Check sheet for the modelled part. Datum: model origin and axes. Units: mm. A direction names the side the tool comes from. Give positions to 0.01 mm unless a question says otherwise; leave off trailing zeros. Loops run counter-clockwise (first coordinate to the right, second up) from the corner with the lowest first, then second, coordinate; pieces in that order, holes last.
```python
from build123d import *

# Parameters (mm, degrees)
SKETCH1_W                    = 106
SKETCH1_H                    = 814
BASE_FLANGE1_DEPTH           = 1
EDGE_FLANGE1_STRIP_W         = 6
EDGE_FLANGE1_STRIP_H         = 1
EDGE_FLANGE1_STRIP_CUT_DEPTH = 814
EDGE_FLANGE1_DEPTH           = 814
EDGE_FLANGE2_STRIP_W         = 6
EDGE_FLANGE2_STRIP_H         = 1
EDGE_FLANGE2_STRIP_CUT_DEPTH = 814
EDGE_FLANGE2_DEPTH           = 814
EDGE_FLANGE4_STRIP_W         = 6
EDGE_FLANGE4_STRIP_H         = 1
EDGE_FLANGE4_STRIP_CUT_DEPTH = 814
EDGE_FLANGE4_DEPTH           = 814
SKETCH19_R                   = 3
CUT_EXTRUDE2_DEPTH           = 10


# Sheet-metal steps are written as plain solids
with BuildPart() as part:
    # Sketch1 → Base-Flange1 (new body)
    with BuildSketch(Plane(origin=(0, 0, 0), x_dir=(1, 0, 0), z_dir=(0, 1, 0))):
        with Locations((53, 407)):
            Rectangle(SKETCH1_W, SKETCH1_H)
    extrude(amount=-BASE_FLANGE1_DEPTH)

    # Edge-Flange1 strip (across the edge) → Edge-Flange1 strip cut (cut)
    with BuildSketch(Plane(origin=(106, 0, 0), x_dir=(-1, 0, 0), z_dir=(0, 0, -1))):
        with Locations((-1, -0.5)):
            Rectangle(EDGE_FLANGE1_STRIP_W, EDGE_FLANGE1_STRIP_H)
    extrude(amount=EDGE_FLANGE1_STRIP_CUT_DEPTH, mode=Mode.SUBTRACT)

    # Edge-Flange1 section (across the edge) → Edge-Flange1 (add)
    with BuildSketch(Plane(origin=(106, 0, 0), x_dir=(-1, 0, 0), z_dir=(0, 0, -1))):
        with BuildLine():
            Line((0, 1), (0, 19))
            Line((0, 19), (1, 19))
            Line((1, 19), (1, 1))
            ThreePointArc((1, 1), (1.292893219, 0.292893219), (2, 0))
            Line((2, 0), (2, -1))
            ThreePointArc((2, -1), (0.585786438, -0.414213562), (0, 1))
        make_face()
    extrude(amount=EDGE_FLANGE1_DEPTH)

    # Edge-Flange2 strip (across the edge) → Edge-Flange2 strip cut (cut)
    with BuildSketch(Plane(origin=(105, 19, 0), x_dir=(0, -1, 0), z_dir=(0, 0, -1))):
        with Locations((-1, -0.5)):
            Rectangle(EDGE_FLANGE2_STRIP_W, EDGE_FLANGE2_STRIP_H)
    extrude(amount=EDGE_FLANGE2_STRIP_CUT_DEPTH, mode=Mode.SUBTRACT)

    # Edge-Flange2 section (across the edge) → Edge-Flange2 (add)
    with BuildSketch(Plane(origin=(105, 19, 0), x_dir=(0, -1, 0), z_dir=(0, 0, -1))):
        with BuildLine():
            Line((0, 1), (0, 18))
            Line((0, 18), (1, 18))
            Line((1, 18), (1, 1))
            ThreePointArc((1, 1), (1.292893219, 0.292893219), (2, 0))
            Line((2, 0), (2, -1))
            ThreePointArc((2, -1), (0.585786438, -0.414213562), (0, 1))
        make_face()
    extrude(amount=EDGE_FLANGE2_DEPTH)

    # Edge-Flange4 strip (across the edge) → Edge-Flange4 strip cut (cut)
    with BuildSketch(Plane.XY.offset(-814)):
        with Locations((-1, -0.5)):
            Rectangle(EDGE_FLANGE4_STRIP_W, EDGE_FLANGE4_STRIP_H)
    extrude(amount=EDGE_FLANGE4_STRIP_CUT_DEPTH, mode=Mode.SUBTRACT)

    # Edge-Flange4 section (across the edge) → Edge-Flange4 (add)
    with BuildSketch(Plane.XY.offset(-814)):
        with BuildLine():
            Line((0, 1), (0, 41))
            Line((0, 41), (1, 41))
            Line((1, 41), (1, 1))
            ThreePointArc((1, 1), (1.292893219, 0.292893219), (2, 0))
            Line((2, 0), (2, -1))
            ThreePointArc((2, -1), (0.585786438, -0.414213562), (0, 1))
        make_face()
    extrude(amount=EDGE_FLANGE4_DEPTH)

    # Sketch19 → Cut-Extrude2 (cut)
    with BuildSketch(Plane(origin=(0, 19, 0), x_dir=(1, 0, 0), z_dir=(0, 1, 0))):
        with Locations(Location((93, 751, 0), (0, 0, 180))):
            Circle(SKETCH19_R)
        with Locations(Location((93, 706, 0), (0, 0, 180))):
            Circle(SKETCH19_R)
        with Locations(Location((93, 538, 0), (0, 0, 180))):
            Circle(SKETCH19_R)
        with Locations(Location((93, 370, 0), (0, 0, 180))):
            Circle(SKETCH19_R)
        with Locations(Location((93, 202, 0), (0, 0, 180))):
            Circle(SKETCH19_R)
        with Locations(Location((93, 34, 0), (0, 0, 180))):
            Circle(SKETCH19_R)
    extrude(amount=-CUT_EXTRUDE2_DEPTH, mode=Mode.SUBTRACT)


solid = part.part
```
(1) Section check A-A on z = -496. Record the boundary of the cut face in (x, y).
(2) Section check B-B on x = 65.5. Record the boundary of the cut face in (y, z).
(3) Gauge pin test, flat ends, axial feed: pin 1 Ø4 at (x, z) = (23.5, -103) entering from +Y; pin 2 Ø18.5 at (x, z) = (93, -418) entering from +Y; pin 3 Ø8 at (y, z) = (21.5, -143.5) entering from +X. Record the tip position at first contact, or that the pin passes through.
(4) Material ranges on line 1 (X direction, y = 18.8, z = -202); line 2 (X direction, y = 16, z = -685); line 3 (Y direction, x = 92.5, z = -59), recorded low to high.
(5) Access from +Z, -Z, +X, -X, +Y, -Y to the whole of each face (thin tool, end or side, straight path). Record for faces 1 (the face through (1, 21, -413)), 2 (the face through (105, 9, -401)), 3 (the face through (106, 9, -401)).
(6) Release check for a two-part mould opening along Y. For faces 4 (the face through (96, 19, -401)), 5 (the face through (95, 18, -401)), 6 (the face through (0, 21, -413)), 7 (the face through (52, -1, -413)) record: pulls with the +Y half, pulls with the -Y half, needs draft (parallel to the pull), parting line crosses it, or undercut.
Computed values:
1. outline: (0, 1) arc R2 ccw to (2, -1) - (104, -1) arc R2 ccw to (106, 1) - (106, 17) arc R2 ccw to (104, 19) - (87, 19) - (87, 18) - (104, 18) arc R1 cw to (105, 17) - (105, 1) arc R1 cw to (104, 0) - (2, 0) arc R1 cw to (1, 1) - (1, 41) - (0, 41) - close
2. outline: (-1, -814) - (0, -814) - (0, 0) - (-1, 0) - close
3. pin 1: stops at y = 0
3. pin 2: stops at y = 19
3. pin 3: stops at x = 105.94
4. line 1: x = 0 to 1, 87 to 90, 96 to 104.87
4. line 2: x = 0 to 1, 105 to 106
4. line 3: y = -1 to 0, 18 to 19
5. face 1: +Z, -Z, +Y
5. face 2: +Z, -Z
5. face 3: +Z, -Z, +X, +Y, -Y
6. face 4: pulls with the +Y half
6. face 5: undercut
6. face 6: needs draft
6. face 7: pulls with the -Y half
